Geometry: final body of the model. Coordinates: model frame, mm. A direction names the side the tool comes from. Round coordinates to 2 decimals unless told otherwise and drop trailing zeros. Write each loop counter-clockwise with the first axis right and the second up, starting at its lowest first coordinate (ties: lowest second). Pieces come first, ordered by that corner, then holes. Notation, with made-up numbers: (-37.75, -22) - (-1.75, -22) arc R26 ccw to (-1.75, 3) - close; hole circle Ø5 at (54, 9). An arc over 180 degrees is marked (long way). Use a Markdown table: item, result. Add a question column.
```python
from build123d import *

# Parameters (mm, degrees)
F3_R = 5


with BuildPart() as f2:
    # F0 (on Front) → F2 (revolve)
    with BuildSketch(Plane.XZ):
        Polygon((-7.5, 0), (-5, 0), (-11.994615, 15), (-15.744615, 15), (-10.972315, 4.765769), (-32.048318, 4.765769), (-30.991772, 2.5), (-8.665769, 2.5), align=None)
    revolve(axis=Axis((0, 0, 12.728581), (0, 0, 1)))

    # F3
    f3_edges = [f2.edges().sort_by_distance(p)[0] for p in [
        (10.972315, 0, 4.765769),
    ]]
    fillet(f3_edges, radius=F3_R)


solid = f2.part
```
1) Pin query (flat end, axial travel): P1, Ø6, axis at x = -1.5, z = 7.5, coming from the +Y side; P2, Ø2, axis at x = -15.5, z = 11.5, coming from the -Y side; P3, Ø8, axis at y = -3, z = 12, coming from the -X side; P4, Ø12, axis at x = 19, y = -20.5, coming from the -Z side. Return the tip coordinate at first contact, or that it passes through.
2) Draft query along Y for faces 1 (the conical face through (1.516, 6.826, 4.272)), 2 (the conical face through (1.869, -14.238, 12.03)), 3 (the flat face through (-6.5, 6.5, 2.5)). Return one class per face: released by +Y, released by -Y, zero draft, split by the parting line, or undercut.
3) Set-up query: faces 4 (the flat face through (-4, 12, 15)), 5 (the flat face through (14, 14, 4.766)). Return all of +Z, -Z, +X, -X, +Y, -Y with unobstructed straight access to the full face (end or side cutting, diameter ignored); none if empty.
4) Material intervals for L1, parallel to Z at x = 8.5, y = -17; L2, parallel to X at y = -3.5, z = 3; L3, parallel to X at y = 0, z = 5.25, sorted ascending. Write a range as from..to.
5) Section C-C, the plane z = 4. Return the cut outline in (x, y), then the cut area to 3 significant figures.
6) Section A-A, the plane x = 0. Return the cut outline in (y, z), then the cut area to 3 significant figures.
7) Section D-D, the plane z = 12.75. Return the cut outline in (x, y), then the cut area to 3 significant figures.
Output values:
| question | item | result |
|---|---|---|
| 1 | P1 | stops at y = 32.05 |
| 1 | P2 | passes through |
| 1 | P3 | stops at x = -15.74 |
| 1 | P4 | stops at z = 2.5 |
| 2 | face 1 | undercut |
| 2 | face 2 | split by the parting line |
| 2 | face 3 | zero draft |
| 3 | face 4 | +Z, +X, -X, +Y, -Y |
| 3 | face 5 | +Z |
| 4 | L1 | z = 2.5..4.77 |
| 4 | L2 | x = -31.03..-5.36, 5.36..31.03 |
| 4 | L3 | x = -16.67..-7.45, 7.45..16.67 |
| 5 | outline | circle Ø63.38 at (0, 0); hole circle Ø13.73 at (0, 0) |
| 5 | area | 3,010 mm^2 |
| 6 | outline | (-32.05, 4.77) - (-30.99, 2.5) - (-8.67, 2.5) - (-7.5, 0) - (-5, 0) - (-11.99, 15) - (-15.74, 15) - (-14.29, 11.88) arc R5 cw to (-18.82, 4.77) - close; (5, 0) - (7.5, 0) - (8.67, 2.5) - (30.99, 2.5) - (32.05, 4.77) - (18.82, 4.77) arc R5 cw to (14.29, 11.88) - (15.74, 15) - (11.99, 15) - close |
| 6 | area | 230 mm^2 |
| 7 | outline | circle Ø29.39 at (0, 0); hole circle Ø21.89 at (0, 0) |
| 7 | area | 302 mm^2 |
